Source: three-view drawing plus pictorial views. Frame: mm from the lowest corner of the part. A direction names the side the tool comes from. Give positions to 0.01 mm unless a question says otherwise; leave off trailing zeros. Loops run counter-clockwise (first coordinate to the right, second up) from the corner with the lowest first, then second, coordinate; pieces in that order, holes last.
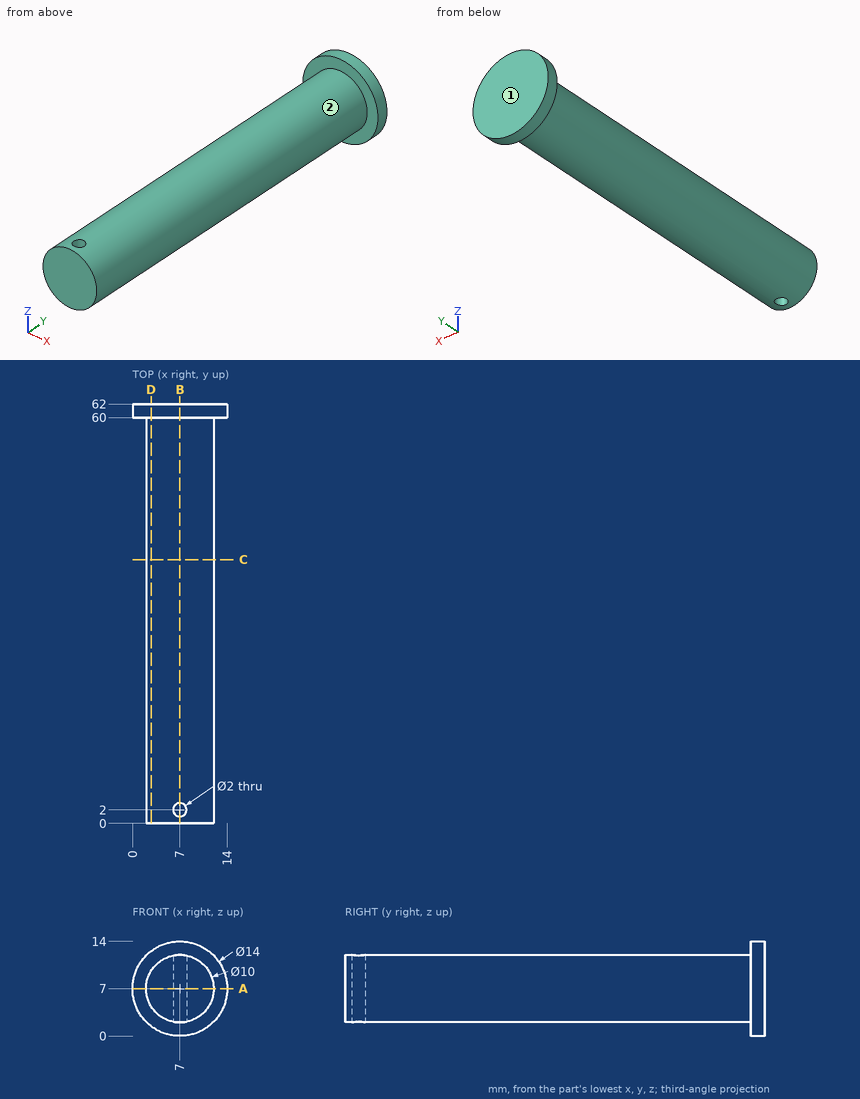
Q1. Section query B-B, the plane x = 7. Return loops of the section in (y, z), and give its area (3 significant figures).
Q2. Section query C-C, the plane y = 39. Return loops of the section in (x, z), and give its area (3 significant figures).
Q3. Section query A-A, the plane z = 7. Return loops of the section in (x, y), and give its area (3 significant figures).
Q4. Material intervals for probe 1 along Y at (x, z) = (7, 7); probe 2 along Y at (x, z) = (1, 4.25); probe 3 along Z at (x, y) = (6.75, 14.5), sorted ascending.
Q5. Pin query (flat end, axial travel): pin 1 Ø4 at (y, z) = (27, 4) entering from -X; pin 2 Ø1.2 at (x, y) = (7, 2) entering from -Z; pin 3 Ø2 at (x, y) = (3, 38) entering from -Z; pin 4 Ø1 at (x, y) = (6.5, 17.5) entering from +Z. Return the tip coordinate at first contact, or that it passes through.
Q6. Reachability of the marked faces 1 and 2 from +Z, -Z, +X, -X, +Y, -Y: full face, straight path, thin tool, end or side. Return the list, or none.
Q7. Section query D-D, the plane x = 2.75. Return loops of the section in (y, z), and give its area (3 significant figures).
Resolved:
1. outline: (0, 2) - (1, 2) - (1, 12) - (0, 12) - close; (3, 2) - (60, 2) - (60, 0) - (62, 0) - (62, 14) - (60, 14) - (60, 12) - (3, 12) - close
1. area: 608 mm2
2. outline: circle Ø10 at (7, 7)
2. area: 78.5 mm2
3. outline: (0, 60) - (2, 60) - (2, 0) - (12, 0) - (12, 60) - (14, 60) - (14, 62) - (0, 62) - close; hole circle Ø2 at (7, 2)
3. area: 625 mm2
4. probe 1: y = 0 to 1, 3 to 62
4. probe 2: y = 60 to 62
4. probe 3: z = 2.01 to 11.99
5. pin 1: stops at x = 2.1
5. pin 2: passes through
5. pin 3: stops at z = 3
5. pin 4: stops at z = 12
6. face 1: +Z, -Z, +X, -X, +Y
6. face 2: -Y
7. outline: (0, 4.37) - (60, 4.37) - (60, 1.44) - (62, 1.44) - (62, 12.56) - (60, 12.56) - (60, 9.63) - (0, 9.63) - close
7. area: 338 mm2
